```python
from build123d import *

# Parameters (mm, degrees)
BOX007_W               = 100
BOX007_H               = 100
BOX007_DEPTH           = 100
BOX007_PLACEMENT_ANGLE = 135
BOX006_W               = 200
BOX006_H               = 100
BOX006_DEPTH           = 100
BOX006_PLACEMENT_ANGLE = 135
BOX005_W               = 100
BOX005_H               = 100
BOX005_DEPTH           = 100
BOX004_W               = 20
BOX004_H               = 20
BOX004_DEPTH           = 80
BOX003_W               = 20
BOX003_H               = 20
BOX003_DEPTH           = 80
BOX002_W               = 10
BOX002_H               = 25
BOX002_DEPTH           = 35
BOX002_PITCH_ANGLE     = -15
BOX001_W               = 10
BOX001_H               = 25
BOX001_DEPTH           = 35
BOX001_PITCH_ANGLE     = 15
BOX_W                  = 20
BOX_H                  = 25
BOX_DEPTH              = 35
CYLINDER005_R          = 10
CYLINDER005_DEPTH      = 180
CYLINDER005_ROLL_ANGLE = 90
CYLINDER004_R          = 54
CYLINDER004_DEPTH      = 100
CYLINDER003_R          = 59
CYLINDER003_DEPTH      = 10
CYLINDER002_R          = 64
CYLINDER002_DEPTH      = 85
CYLINDER001_R          = 70
CYLINDER001_DEPTH      = 90
CYLINDER_R             = 80
CYLINDER_DEPTH         = 10
FILLET_R               = 3
FILLET001_R            = 5
FILLET002_R            = 5
CUT009_ROLL_ANGLE      = 90
CUT009_PITCH_ANGLE     = -45
CUT009_PLACEMENT_ANGLE = -45


with BuildPart() as cube004:
    # Box007 → Box007 (new body)
    with BuildSketch(Plane.XY):
        with Locations((50, 50)):
            Rectangle(BOX007_W, BOX007_H)
    extrude(amount=BOX007_DEPTH)


with BuildPart() as cube004_1:
    # Box007 placement: moved
    add(cube004.part.rotate(Axis((0, 0, 0), (0, 0, -1)), BOX007_PLACEMENT_ANGLE))


with BuildPart() as cube003:
    # Box006 → Box006 (new body)
    with BuildSketch(Plane.XY):
        with Locations((100, 50)):
            Rectangle(BOX006_W, BOX006_H)
    extrude(amount=BOX006_DEPTH)


with BuildPart() as cube003_1:
    # Box006 placement: moved
    add(cube003.part.moved(Location((71, -71, 0))).rotate(Axis((71, -71, 0), (0, 0, 1)), BOX006_PLACEMENT_ANGLE))


with BuildPart() as cube002:
    # Box005 → Box005 (new body)
    with BuildSketch(Plane.XY):
        with Locations((50, 50)):
            Rectangle(BOX005_W, BOX005_H)
    extrude(amount=BOX005_DEPTH)


with BuildPart() as tab_cut_l:
    # Box004 → Box004 (new body)
    with BuildSketch(Plane(origin=(-83, -10, 20), x_dir=(1, 0, 0), z_dir=(0, 0, 1))):
        with Locations((10, 10)):
            Rectangle(BOX004_W, BOX004_H)
    extrude(amount=BOX004_DEPTH)


with BuildPart() as tab_cut_r:
    # Box003 → Box003 (new body)
    with BuildSketch(Plane(origin=(63, -10, 20), x_dir=(1, 0, 0), z_dir=(0, 0, 1))):
        with Locations((10, 10)):
            Rectangle(BOX003_W, BOX003_H)
    extrude(amount=BOX003_DEPTH)


with BuildPart() as cube001:
    # Box002 → Box002 (new body)
    with BuildSketch(Plane.XY):
        with Locations((5, 12.5)):
            Rectangle(BOX002_W, BOX002_H)
    extrude(amount=BOX002_DEPTH)


with BuildPart() as cube001_1:
    # Box002 pitch: moved
    add(cube001.part.rotate(Axis((0, 0, 0), (0, 1, 0)), BOX002_PITCH_ANGLE))


with BuildPart() as cube001_2:
    # Box002 placement: moved
    add(cube001_1.part.moved(Location((-9.95, 48, 64))))


with BuildPart() as cube:
    # Box001 → Box001 (new body)
    with BuildSketch(Plane.XY):
        with Locations((5, 12.5)):
            Rectangle(BOX001_W, BOX001_H)
    extrude(amount=BOX001_DEPTH)


with BuildPart() as cube_1:
    # Box001 pitch: moved
    add(cube.part.rotate(Axis((0, 0, 0), (0, 1, 0)), BOX001_PITCH_ANGLE))


with BuildPart() as cube_2:
    # Box001 placement: moved
    add(cube_1.part.moved(Location((0, 48, 65))))


with BuildPart() as bearing_slot:
    # Box → Box (new body)
    with BuildSketch(Plane(origin=(-10, 48, 65), x_dir=(1, 0, 0), z_dir=(0, 0, 1))):
        with Locations((10, 12.5)):
            Rectangle(BOX_W, BOX_H)
    extrude(amount=BOX_DEPTH)


with BuildPart() as bearing_holes:
    # Cylinder005 → Cylinder005 (new body)
    with BuildSketch(Plane.XY):
        Circle(CYLINDER005_R)
    extrude(amount=CYLINDER005_DEPTH)


with BuildPart() as bearing_holes_1:
    # Cylinder005 roll: moved
    add(bearing_holes.part.rotate(Axis((0, 0, 0), (1, 0, 0)), CYLINDER005_ROLL_ANGLE))


with BuildPart() as bearing_holes_2:
    # Cylinder005 placement: moved
    add(bearing_holes_1.part.moved(Location((0, 90, 65))))


with BuildPart() as through_hole:
    # Cylinder004 → Cylinder004 (new body)
    with BuildSketch(Plane.XY):
        Circle(CYLINDER004_R)
    extrude(amount=CYLINDER004_DEPTH)


with BuildPart() as inner_lip:
    # Cylinder003 → Cylinder003 (new body)
    with BuildSketch(Plane.XY.offset(80)):
        Circle(CYLINDER003_R)
    extrude(amount=CYLINDER003_DEPTH)


with BuildPart() as inner_hole:
    # Cylinder002 → Cylinder002 (new body)
    with BuildSketch(Plane.XY):
        Circle(CYLINDER002_R)
    extrude(amount=CYLINDER002_DEPTH)


with BuildPart() as body_cylinder:
    # Cylinder001 → Cylinder001 (new body)
    with BuildSketch(Plane.XY.offset(5)):
        Circle(CYLINDER001_R)
    extrude(amount=CYLINDER001_DEPTH)


with BuildPart() as cut010:
    # Cylinder → Cylinder (new body)
    with BuildSketch(Plane.XY):
        Circle(CYLINDER_R)
    extrude(amount=CYLINDER_DEPTH)

    # Fusion: union Body_Cylinder
    add(body_cylinder.part)

    # Cut: cut Inner_Hole
    add(inner_hole.part, mode=Mode.SUBTRACT)

    # Fusion001: union Inner_Lip
    add(inner_lip.part)

    # Cut001: cut Through_Hole
    add(through_hole.part, mode=Mode.SUBTRACT)

    # Fillet
    fillet_edges = [cut010.edges().sort_by_distance(p)[0] for p in [
        (-70, 0, 10),
    ]]
    fillet(fillet_edges, radius=FILLET_R)

    # Fillet001
    fillet001_edges = [cut010.edges().sort_by_distance(p)[0] for p in [
        (-80, 0, 0),
    ]]
    fillet(fillet001_edges, radius=FILLET001_R)

    # Fillet002
    fillet002_edges = [cut010.edges().sort_by_distance(p)[0] for p in [
        (-70, 0, 95),
    ]]
    fillet(fillet002_edges, radius=FILLET002_R)

    # Cut002: cut Bearing_Holes
    add(bearing_holes_2.part, mode=Mode.SUBTRACT)

    # Cut003: cut Bearing_Slot
    add(bearing_slot.part, mode=Mode.SUBTRACT)

    # Cut004: cut Cube
    add(cube_2.part, mode=Mode.SUBTRACT)

    # Cut005: cut Cube001
    add(cube001_2.part, mode=Mode.SUBTRACT)

    # Cut006: cut Tab_Cut_R
    add(tab_cut_r.part, mode=Mode.SUBTRACT)

    # Cut007: cut Tab_Cut_L
    add(tab_cut_l.part, mode=Mode.SUBTRACT)

    # Cut008: cut Cube002
    add(cube002.part, mode=Mode.SUBTRACT)

    # Cut009: cut Cube003
    add(cube003_1.part, mode=Mode.SUBTRACT)


with BuildPart() as cut010_1:
    # Cut009 roll: moved
    add(cut010.part.rotate(Axis((0, 0, 0), (1, 0, 0)), CUT009_ROLL_ANGLE))


with BuildPart() as cut010_2:
    # Cut009 pitch: moved
    add(cut010_1.part.rotate(Axis((0, 0, 0), (0, 1, 0)), CUT009_PITCH_ANGLE))


with BuildPart() as cut010_3:
    # Cut009 placement: moved
    add(cut010_2.part.rotate(Axis((0, 0, 0), (0, 0, 1)), CUT009_PLACEMENT_ANGLE))

    # Cut010: cut Cube004
    add(cube004_1.part, mode=Mode.SUBTRACT)


solid = cut010_3.part
```
Read the model definition and answer for the solid it produces. Units are mm, in the model's axes. A direction names the side the tool comes from. Coordinates: 2 decimals unless noted, no trailing zeros. Answer in a Markdown table with one row per item.
1. Straight lines are drawn through the part: line 1 (Y direction, x = -102, z = 3); line 2 (X direction, y = -18, z = 24.5); line 3 (X direction, y = 3.5, z = 45.5). For each, find the intervals that lie inside material, in ascending order.
Conclusion:
| item | result |
|---|---|
| line 1 | y = -25.75 to -18.21, -11.59 to -3.1 |
| line 2 | x = -110.6 to -101.62 |
| line 3 | x = -71.73 to -60.85 |
2. Determine the mould class of faces 1 (the face through (-81, 14, 0)), 2 (the face through (-108.55, -25.8, 12.83)), 3 (the face through (-98.47, -18.16, 16)), 4 (the face through (-77.488, -4.046, 42.337)) for opening direction X: +X half, -X half, draft (parallel to the pull), parting line (faces both ways), or undercut.
Conclusion:
| item | result |
|---|---|
| face 1 | draft |
| face 2 | -X half |
| face 3 | undercut |
| face 4 | undercut |
3. Given pin 1 (10 mm diameter, centred on y = -14.5, z = 31, fed in from -X); pin 2 (6 mm diameter, centred on x = -93, z = 6.5, fed in from -Y); pin 3 (10 mm diameter, centred on y = 37, z = 8, fed in from +X), each flat-ended and moving along its own axis, determine where each tip first touches the part or whether it passes through.
Conclusion:
| item | result |
|---|---|
| pin 1 | stops at x = -109.22 |
| pin 2 | stops at y = -20.24 |
| pin 3 | stops at x = -47.71 |
4. Which of the six approach directions +Z, -Z, +X, -X, +Y, -Y give full straight-line access (tool end or side, diameter ignored) to faces 5 (the face through (-56.32, 42.18, 29.46)), 6 (the face through (-102.07, -18.14, 16.24)), 7 (the face through (-49.018, 19.314, 48.318)), 8 (the face through (-95.178, -17.959, 14.945))?
Conclusion:
| item | result |
|---|---|
| face 5 | +Z, -X |
| face 6 | none |
| face 7 | +Z, +X, -Y |
| face 8 | -Z, +X |
